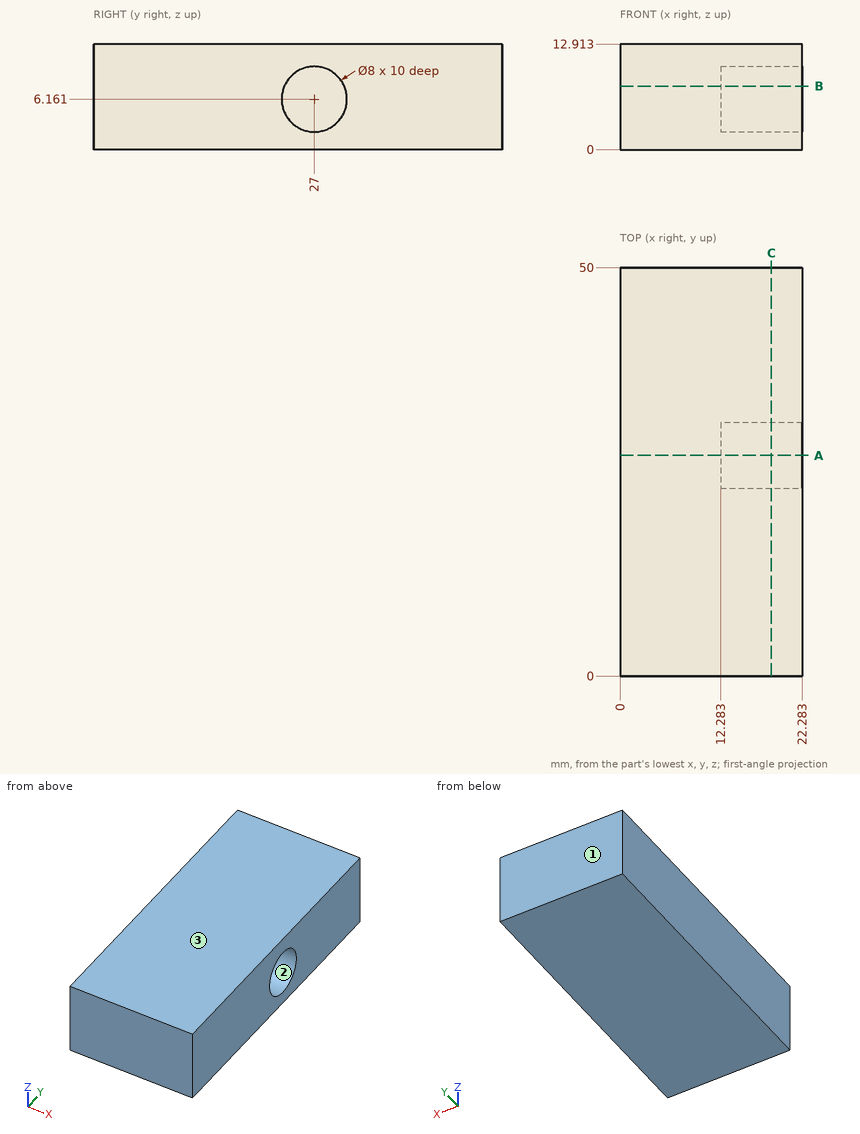
Geometry check sheet. Reference: drawing and pictorial views, mm from the part's lowest x, y, z. Round coordinates to 2 decimals unless told otherwise and drop trailing zeros. Loops run counter-clockwise (first coordinate to the right, second up) from the corner with the lowest first, then second, coordinate; pieces in that order, holes last. Notation, with made-up numbers: (73.5, 68.25) - (83.5, 68.25) arc R32 ccw to (83.5, 101.25) - close; hole circle Ø8 at (29.25, -25.5). An arc over 180 degrees is marked (long way). Answer in a Markdown table with one row per item. Add a question column.
Q1. Material ranges on line 1 (Z direction, x = 16.25, y = 27); line 2 (Y direction, x = 12.75, z = 6); line 3 (X direction, y = 24.5, z = 9.25), recorded low to high.
Q2. Section check A-A on y = 27. Enter the section's corners in (x, z), plus the area to 3 significant figures.
Q3. Section check B-B on z = 7.75. Enter the section's corners in (x, y), plus the area to 3 significant figures.
Q4. Section check C-C on x = 18.5. Enter the section's corners in (y, z).
Q5. Release check for a two-part mould opening along Y. For the marked faces 1, 2 and 3 record: pulls with the +Y half, pulls with the -Y half, needs draft (parallel to the pull), parting line crosses it, or undercut.
Found:
| question | item | result |
|---|---|---|
| 1 | line 1 | z = 0 to 2.16, 10.16 to 12.91 |
| 1 | line 2 | y = 0 to 23, 31 to 50 |
| 1 | line 3 | x = 0 to 12.28 |
| 2 | outline | (0, 0) - (22.28, 0) - (22.28, 2.16) - (12.28, 2.16) - (12.28, 10.16) - (22.28, 10.16) - (22.28, 12.91) - (0, 12.91) - close |
| 2 | area | 208 mm² |
| 3 | outline | (0, 0) - (22.28, 0) - (22.28, 23.33) - (12.28, 23.33) - (12.28, 30.67) - (22.28, 30.67) - (22.28, 50) - (0, 50) - close |
| 3 | area | 1,040 mm² |
| 4 | outline | (0, 0) - (50, 0) - (50, 12.91) - (0, 12.91) - close; hole circle Ø8 at (27, 6.16) |
| 5 | face 1 | pulls with the +Y half |
| 5 | face 2 | undercut |
| 5 | face 3 | needs draft |
